from build123d import *

# Parameters (mm, degrees)
F0_R     = 13.65
F0_R_2   = 6.35
F1_DEPTH = 15
F2_W     = 120
F2_H     = 40
F3_DEPTH = 7
F5_D     = 9
F7_D     = 10
F7_DEPTH = 100
F7_TIP   = 3.0043030951


# Not quite as in the source:
# - a pattern or mirror of a feature is missing from the dataset's text; its kind, count and spacing are read off the source's solid


with BuildPart() as f1:
    # F0 (on Front) → F1 (new body)
    with BuildSketch(Plane.XZ):
        Circle(F0_R)
        Circle(F0_R_2, mode=Mode.SUBTRACT)
    extrude(amount=F1_DEPTH)

    # F2 (on Front) → F3 (join)
    with BuildSketch(Plane.XZ):
        Rectangle(F2_W, F2_H)
    extrude(amount=-F3_DEPTH)

    # F5 (through all)
    with Locations(Plane.XZ):
        with Locations((-47.5, 10), (-47.5, -10)):
            f5 = Hole(F5_D / 2)

    # F5_copies: F5 across plane
    add(f5.mirror(Plane(origin=(0, 0, 0), x_dir=(0, 0, 1), z_dir=(1, 0, 0))), mode=Mode.SUBTRACT)

    # F7
    with Locations(Plane(origin=(0, 7, 0), x_dir=(-1, 0, 0), z_dir=(0, 1, 0))):
        with Locations((0, 0)):
            Hole(F7_D / 2, depth=F7_DEPTH)
            with Locations((0, 0, -(F7_DEPTH + F7_TIP / 2))):  # 118° drill point
                Cone(0, F7_D / 2, F7_TIP, mode=Mode.SUBTRACT)


solid = f1.part
Input: part model. Units: mm. Frame: model coordinates. A direction names the side the tool comes from. Give positions to 0.01 mm unless a question says otherwise; leave off trailing zeros. Write each loop counter-clockwise with the first axis right and the second up, starting at its lowest first coordinate (ties: lowest second). Pieces come first, ordered by that corner, then holes.
Q1. Section D-D, the plane y = -1.75. Output: boundary loops of the cut face in (x, z).
Q2. Section C-C, the plane x = 0. Output: boundary loops of the cut face in (y, z), plus the area to 3 significant figures.
Q3. Pull-direction query (X, two-part tool) for faces 3 (the face through (-14, 0, 0)), 4 (the face through (-51.792, 3.549, 11.352)), 5 (the face through (2, 0, -5)), 6 (the face through (60, 3, 0)); classes: pulls with the +X half, pulls with the -X half, needs draft (parallel to the pull), parting line crosses it, or undercut.
Q4. Section A-A, the plane x = 47.5. Output: boundary loops of the cut face in (y, z).
Q5. Material intervals for probe 1 along Z at (x, y) = (-47.5, 4.5); probe 2 along Z at (x, y) = (0, -5); probe 3 along X at (y, z) = (-6.25, -12.5), sorted ascending.
Q6. Set-up query: faces 1 (the face through (-10.83, -7.4, -8.31)), 2 (the face through (-1, 7, 9)). Return all of +Z, -Z, +X, -X, +Y, -Y with unobstructed straight access to the full face (end or side cutting, diameter ignored); none if empty.
Q7. First-contact query: P1, Ø8, axis at y = -12, z = 4, coming from the -X side; P2, Ø4, axis at y = -3.5, z = -13.5, coming from the -X side; P3, Ø14.5, axis at x = 47.5, z = 10, coming from the -Y side. Flat tips, straight axial feed; report the tip coordinate or a pass-through.
Q8. Section B-B, the plane z = 0. Output: boundary loops of the cut face in (x, y), plus the area to 3 significant figures.
Filled in:
1. outline: circle Ø27.3 at (0, 0); hole circle Ø12.7 at (0, 0)
2. outline: (-15, -13.65) - (0, -13.65) - (0, -20) - (7, -20) - (7, -5) - (0, -5) - (0, -6.35) - (-15, -6.35) - close; (-15, 6.35) - (0, 6.35) - (0, 5) - (7, 5) - (7, 20) - (0, 20) - (0, 13.65) - (-15, 13.65) - close
2. area: 429 mm2
3. face 3: needs draft
3. face 4: undercut
3. face 5: undercut
3. face 6: pulls with the +X half
4. outline: (0, -20) - (7, -20) - (7, -14.5) - (0, -14.5) - close; (0, -5.5) - (7, -5.5) - (7, 5.5) - (0, 5.5) - close; (0, 14.5) - (7, 14.5) - (7, 20) - (0, 20) - close
5. probe 1: z = -20 to -14.5, -5.5 to 5.5, 14.5 to 20
5. probe 2: z = -13.65 to -6.35, 6.35 to 13.65
5. probe 3: x = -5.48 to 5.48
6. face 1: -Y
6. face 2: +Z, -Z, +X, -X, +Y
7. P1: stops at x = -13.65
7. P2: stops at x = -7.35
7. P3: stops at y = 0
8. outline: (-60, 0) - (-13.65, 0) - (-13.65, -15) - (-6.35, -15) - (-6.35, 0) - (-5, 0) - (-5, 7) - (-60, 7) - close; (5, 0) - (6.35, 0) - (6.35, -15) - (13.65, -15) - (13.65, 0) - (60, 0) - (60, 7) - (5, 7) - close
8. area: 989 mm2
